```python
from build123d import *

# Parameters (mm, degrees)
SKETCH1_R           = 4
BOSS_EXTRUDE1_DEPTH = 10


with BuildPart() as part:
    # Sketch1 → Boss-Extrude1 (new body)
    with BuildSketch(Plane.XY):
        with BuildLine():
            ThreePointArc((-10.602156333, 5.620879031), (-10.28227962, -6.186657079), (0, -12))
            Line((0, -12), (0.41879396, -11.992689924))
            Line((0.41879396, -11.992689924), (61.391036956, -10.928415464))
            ThreePointArc((61.391036956, -10.928415464), (79.964133291, -8.081963895), (97.110947363, -0.397631709))
            ThreePointArc((97.110947363, -0.397631709), (98.438615507, 5.04350762), (93.024727532, 6.47826087))
            ThreePointArc((93.024727532, 6.47826087), (77.526052275, 0.15529838), (60.926549925, -2))
            Line((60.926549925, -2), (22, -2))
            ThreePointArc((22, -2), (7, 13), (22, 28))
            ThreePointArc((22, 28), (25.895103095, 32.910039494), (20.227651175, 35.58591406))
            ThreePointArc((20.227651175, 35.58591406), (2.455290247, 23.028888484), (-10.602156333, 5.620879031))
        make_face()
        Circle(SKETCH1_R, mode=Mode.SUBTRACT)
    extrude(amount=BOSS_EXTRUDE1_DEPTH)


solid = part.part
```
Part model, mm, in its own coordinate system. A direction names the side the tool comes from. Round coordinates to 2 decimals unless told otherwise and drop trailing zeros. Order: outer loops, then holes, each group sorted by start corner. A loop starts at its lowest first (then second) coordinate and runs counter-clockwise, first axis right, second up. Notation, with made-up numbers: M -7.75,82 L -3.75,82 A21 cw -3.75,114 Z; hole C -31,9 d6. An arc over 180 degrees is marked long. Answer in a Markdown table with one row per item. Add a question column.
Q1. 3-axis set-ups, long thin cutter, end or side, ignore diameter. For faces 1 (the face through (7, 13, 5)), 2 (the face through (79.711, -8.156, 4.93)): which of +Z, -Z, +X, -X, +Y, -Y reach the whole face in a straight line?
Q2. Cut at B-B on x = 25. Give the cut face in (y, z), and give its area (3 significant figures).
Q3. Cut at A-A on z = 6.5. Give the cut face in (x, y), and give its area (3 significant figures).
Q4. Mould opens along Y. For faces 3 (the face through (77.753, 0.216, 4.93)), 4 (the face through (31, -4, 10)), 5 (the face through (-0.867, -3.905, 4.93)), 6 (the face through (-10.37, -6.04, 4.93)) say: +Y half, -Y half, draft (parallel to the pull), parting line (faces both ways), or undercut.
Q5. Wall check: L1, parallel to Y at x = 57.5, z = 4; L2, parallel to Y at x = 72, z = 2.75; L3, parallel to X at y = 32.5, z = 7.5. Give the ranges that are in metal, low to high. Write a range as from..to.
Q6. Cut at C-C on y = 3. Give the cut face in (x, z), and give its area (3 significant figures).
Q7. Pin check, flat tips, straight feed: pin 1 (2 mm diameter, centred on x = 81.5, z = 7.5, fed in from +Y); pin 2 (3 mm diameter, centred on x = 50.5, z = 6, fed in from +Y); pin 3 (3 mm diameter, centred on x = 18, z = 5.5, fed in from +Y). Stop position of each tip, or through.
Q8. Cut at D-D on y = 30. Give the cut face in (x, z), and give its area (3 significant figures).
Established:
| question | item | result |
|---|---|---|
| 1 | face 1 | +Z, -Z |
| 1 | face 2 | +Z, -Z, +X, -Y |
| 2 | outline | M -11.56,0 L -2,0 L -2,10 L -11.56,10 Z; M 29.35,0 L 34.65,0 L 34.65,10 L 29.35,10 Z |
| 2 | area | 149 mm2 |
| 3 | outline | M -10.6,5.62 A12 ccw 0,-12 L 61.39,-10.93 A70 ccw 97.11,-0.4 A4 ccw 93.02,6.48 A65 cw 60.93,-2 L 22,-2 A15 cw 22,28 A4 ccw long 20.23,35.59 A70 ccw Z; hole C 0,0 d8 |
| 3 | area | 1,490 mm2 |
| 4 | face 3 | +Y half |
| 4 | face 4 | draft |
| 4 | face 5 | undercut |
| 4 | face 6 | parting line |
| 5 | L1 | y = -11..-2 |
| 5 | L2 | y = -9.93..-1.05 |
| 5 | L3 | x = 14.64..25.97 |
| 6 | outline | M -11.62,0 L -2.65,0 L -2.65,10 L -11.62,10 Z; M 2.65,0 L 10.82,0 L 10.82,10 L 2.65,10 Z; M 85.93,0 L 99,0 L 99,10 L 85.93,10 Z |
| 6 | area | 302 mm2 |
| 7 | pin 1 | stops at y = 1.68 |
| 7 | pin 2 | stops at y = -2 |
| 7 | pin 3 | stops at y = 35.22 |
| 8 | outline | M 10.85,0 L 25.46,0 L 25.46,10 L 10.85,10 Z |
| 8 | area | 146 mm2 |
